from build123d import *

# Parameters (mm, degrees)
CUT_EXTRUDE1_DEPTH = 1.2
CHAMFER1_SIZE      = 0.3
FILLET1_R          = 0.3


with BuildPart() as part:
    # Sketch1 → Revolve1 (revolve)
    with BuildSketch(Plane(origin=(0, 0, 0), x_dir=(1, 0, 0), z_dir=(0, 1, 0)), mode=Mode.PRIVATE) as revolve1_sk:
        with BuildLine():
            Line((0, 0), (0, 1.5))
            Line((0, 1.5), (12, 1.5))
            Line((12, 1.5), (12, 2.45))
            Line((12, 2.45), (12.7, 2.45))
            add(Edge.make_bspline(
                [(12.7, 2.45), (13.190442748, 2.484618279), (13.5, 1.5)],
                knots=[0, 0, 0, 0.615019669, 0.615019669, 0.615019669], degree=2))
            Line((13.5, 1.5), (13.5, 0))
            Line((13.5, 0), (0, 0))
        make_face()
    revolve(revolve1_sk.sketch.rotate(Axis((-60.710951108, 0, 0), (1, 0, 0)), 180), axis=Axis((-60.710951108, 0, 0), (1, 0, 0)))

    # Sketch2 → Cut-Extrude1 (cut)
    with BuildSketch(Plane(origin=(13.5, 0, 0), x_dir=(0, 0, -1), z_dir=(1, 0, 0))):
        Polygon((0.349309187, 1.095665593), (-0.774219644, 0.850343426), (-1.123528831, -0.245322167), (-0.349309187, -1.095665593), (0.774219644, -0.850343426), (1.123528831, 0.245322167), align=None)
    extrude(amount=-CUT_EXTRUDE1_DEPTH, mode=Mode.SUBTRACT)

    # Chamfer1
    chamfer1_edges = [part.edges().sort_by_distance(p)[0] for p in [
        (0, 0, -1.5),
        (12, 0, -1.5),
    ]]
    chamfer(chamfer1_edges, length=CHAMFER1_SIZE)

    # Fillet1
    fillet1_edges = [part.edges().sort_by_distance(p)[0] for p in [
        (12, 0, -2.45),
    ]]
    fillet(fillet1_edges, radius=FILLET1_R)


solid = part.part
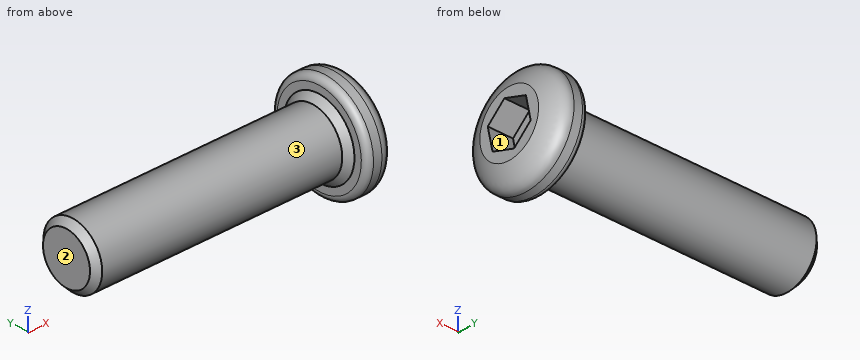
The listing builds one solid part. Answer for the finished solid, in the listing's coordinates (mm). Face numbers are marked on the shaded views. Round coordinates to 2 decimals unless told otherwise and drop trailing zeros. Write each loop counter-clockwise with the first axis right and the second up, starting at its lowest first coordinate (ties: lowest second). Pieces come first, ordered by that corner, then holes. Notation, with made-up numbers: (25.5, 51.25) - (68.5, 51.25) arc R22 cw to (68.5, 78.25) - close; hole circle Ø2 at (68, 6.25). An arc over 180 degrees is marked (long way). Use a Markdown table: item, result. Add a question column.
1. The part is cut by section A-A (x = 8.5). Write down the section's boundary in (y, z).
2. For a pull along Y with two mould halves and no side action, classify the marked faces 1, 2 and 3 as +Y half, -Y half, draft (parallel to the pull), parting line (faces both ways), or undercut.
3. Flat-ended cylindrical pins translate along their axes: P1, Ø1.8, axis at y = 0, z = -0.5, coming from the +X side; P2, Ø1.5, axis at x = 7.5, y = 0, coming from the -Z side; P3, Ø1.5, axis at x = 8.5, y = 2, coming from the +Z side. Find the tip coordinate at first contact, or state that the pin passes through.
4. Consider line 1 (Z direction, x = 3.5, y = 0.9); line 2 (Y direction, x = 2, z = 1.2); line 3 (X direction, y = 1.4, z = 1.45). Determine where each line is inside the solid, lowest interval first.
Reported:
| question | item | result |
|---|---|---|
| 1 | outline | circle Ø3 at (0, 0) |
| 2 | face 1 | undercut |
| 2 | face 2 | draft |
| 2 | face 3 | parting line |
| 3 | P1 | x = 13.5 |
| 3 | P2 | z = -1.5 |
| 3 | P3 | z = 0.83 |
| 4 | line 1 | -1.2 to 1.2 |
| 4 | line 2 | -0.9 to 0.9 |
| 4 | line 3 | 12 to 13.29 |
